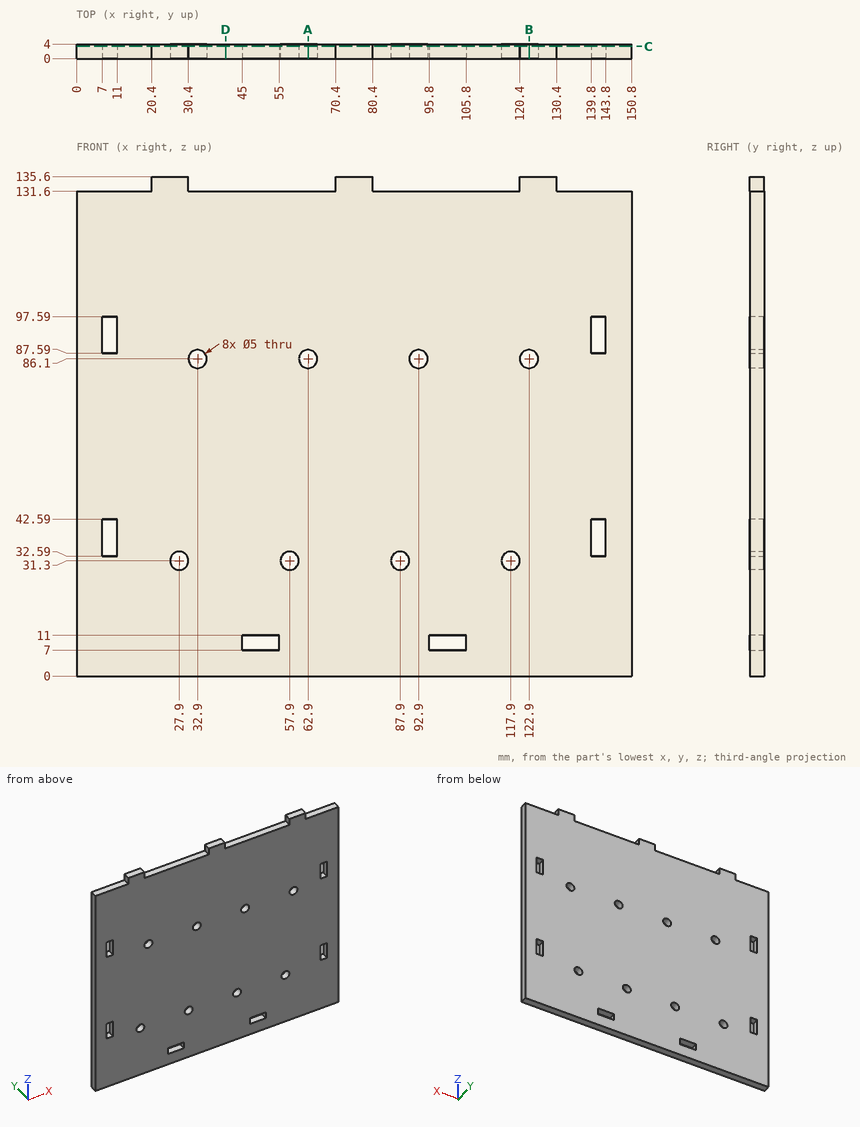
Geometry check sheet. Reference: drawing and pictorial views, mm from the part's lowest x, y, z. Round coordinates to 2 decimals unless told otherwise and drop trailing zeros. Loops run counter-clockwise (first coordinate to the right, second up) from the corner with the lowest first, then second, coordinate; pieces in that order, holes last. Notation, with made-up numbers: (47, 28) - (92, 28) arc R18 ccw to (92, 44) - close; hole circle Ø10 at (-4.75, 0.5). An arc over 180 degrees is marked (long way). One line per question, with ' | ' between items. Start each with the question number.
1. Depth check by flat-ended pin: pin 1 (5 mm diameter, centred on x = 95.5, z = 118.5, fed in from -Y); pin 2 (2 mm diameter, centred on y = 2.5, z = 133, fed in from +X); pin 3 (1.2 mm diameter, centred on x = 141.5, y = 2, fed in from +Z). Enter the tip coordinate at first touch or a pass-through.
2. Cross-section at A-A on x = 62.9. Record the cut outline in (y, z).
3. Scan lines: line 1 (X direction, y = 2.4, z = 93.5); line 2 (Z direction, x = 10, y = 1.4); line 3 (X direction, y = 1.55, z = 31.3). Record each from-to range of solid material in increasing order. Write a range as [from, to].
4. Cross-section at C-C on y = 3.35. State how many separate pieces and enclosed holes the cut face has, then the cut area to 3 significant figures.
5. Cross-section at D-D on x = 40.5. Record the cut outline in (y, z).
6. Cross-section at B-B on x = 122.9. Record the cut outline in (y, z).
Taken from the geometry:
1) pin 1: y = 0 | pin 2: x = 130.4 | pin 3: z = 131.6
2) outline: (0, 0) - (4, 0) - (4, 83.6) - (0, 83.6) - close; (0, 88.6) - (4, 88.6) - (4, 131.6) - (0, 131.6) - close
3) line 1: [0, 7], [11, 139.8], [143.8, 150.8] | line 2: [0, 32.59], [42.59, 87.59], [97.59, 131.6] | line 3: [0, 25.4], [30.4, 55.4], [60.4, 85.4], [90.4, 115.4], [120.4, 150.8]
4) separate pieces: 1 | enclosed holes: 14 | area: 19,600 mm²
5) outline: (0, 0) - (4, 0) - (4, 131.6) - (0, 131.6) - close
6) outline: (0, 0) - (4, 0) - (4, 83.6) - (0, 83.6) - close; (0, 88.6) - (4, 88.6) - (4, 135.6) - (0, 135.6) - close
